Can you work these out from the model? Positions are in its coordinate system, mm. Coordinates: 2 decimals unless noted, no trailing zeros. Loops run counter-clockwise (first coordinate to the right, second up) from the corner with the lowest first, then second, coordinate; pieces in that order, holes last.
```python
from build123d import *

# Parameters (mm, degrees)
BOSS_EXTRU_1_START = -3
ESQUISSE1_R        = 3
BOSS_EXTRU_1_DEPTH = 61
CHANFREIN1_SIZE    = 3.5
CHANFREIN1_SIZE2   = 1.5


with BuildPart() as part:
    # Esquisse1 → Boss.-Extru.1 (new body)
    with BuildSketch(Plane.XY.offset(BOSS_EXTRU_1_START)):
        with Locations(Location((0, 0, 0), (0, 0, 180))):
            Circle(ESQUISSE1_R)
    extrude(amount=BOSS_EXTRU_1_DEPTH)

    # Chanfrein1
    chanfrein1_edges = [part.edges().sort_by_distance(p)[0] for p in [
        (3, 0, 58),
    ]]
    chanfrein1_side = [part.faces().sort_by_distance(p)[0] for p in [
        (3, 0, 27.5),
    ]]
    chamfer(chanfrein1_edges, length=CHANFREIN1_SIZE, length2=CHANFREIN1_SIZE2, reference=chanfrein1_side[0])

    # Esquisse2 → Enlèvement de matière-Révolution1 (revolve, cut)
    with BuildSketch(Plane(origin=(0, 0, 0), x_dir=(1, 0, 0), z_dir=(0, 1, 0))):
        Polygon((-3, 0), (3, 0), (3, 2.5), (2, 1.5), (-2, 1.5), (-3, 2.5), align=None)
    revolve(axis=Axis((-3, 0, 0), (-1, 0, 0)), mode=Mode.SUBTRACT)


solid = part.part
```
Item 1: We'd pull the mould along Z, two halves only. Please class faces 1 (the face through (0.413, 1.861, 57.052)), 2 (the face through (0, 0, -3)), 3 (the face through (-0.03, -0.07, 1.5)): +Z half, -Z half, draft (parallel to the pull), parting line (faces both ways), or undercut.
Results are:
face 1: +Z half
face 2: -Z half
face 3: undercut
Item 2: Suppose I cut it at D-D, the plane z = 20.5. Please give me the cut outline in (x, y).
Results are:
outline: circle Ø6 at (0, 0)
Item 3: Suppose I cut it at A-A, the plane y = 0. Please give me the cut outline in (x, z), plus the area to 3 significant figures.
Results are:
outline: (-3, -3) - (3, -3) - (3, -2.5) - (2, -1.5) - (-2, -1.5) - (-3, -2.5) - close; (-3, 2.5) - (-2, 1.5) - (2, 1.5) - (3, 2.5) - (3, 54.5) - (1.5, 58) - (-1.5, 58) - (-3, 54.5) - close
area: 341 mm2
Item 4: Suppose I cut it at C-C, the plane z = 0. Please give me the cut outline in (x, y), plus the area to 3 significant figures.
Results are:
outline: (-2.36, -1.86) arc R3 ccw to (2.36, -1.86) - (2, -1.5) - (-2, -1.5) - close; (-2.36, 1.86) - (-2, 1.5) - (2, 1.5) - (2.36, 1.86) arc R3 ccw to start
area: 10.6 mm2
Item 5: Suppose I cut it at B-B, the plane x = 0. Please give me the cut outline in (y, z).
Results are:
outline: (-3, -3) - (3, -3) - (3, 54.5) - (1.5, 58) - (-1.5, 58) - (-3, 54.5) - close; hole circle Ø3 at (0, 0)
Item 6: I'm going to push a flat-ended pin straight in: P1, Ø2.5, axis at y = 0, z = 0, coming from the +X side. Where does the tip first touch, or does it pass through?
Results are:
P1: passes through
Item 7: I need wall thicknesses on line 1 along Z through (x, y) = (0.2, 0); line 2 along Z through (x, y) = (0.5, -1.25); line 3 along Y through (x, z) = (-1.2, 0). Which ranges of each line are inside material? Lowest first, please.
Results are:
line 1: z = -3 to -1.5, 1.5 to 58
line 2: z = -3 to -0.83, 0.83 to 58
line 3: y = -2.75 to -1.5, 1.5 to 2.75
